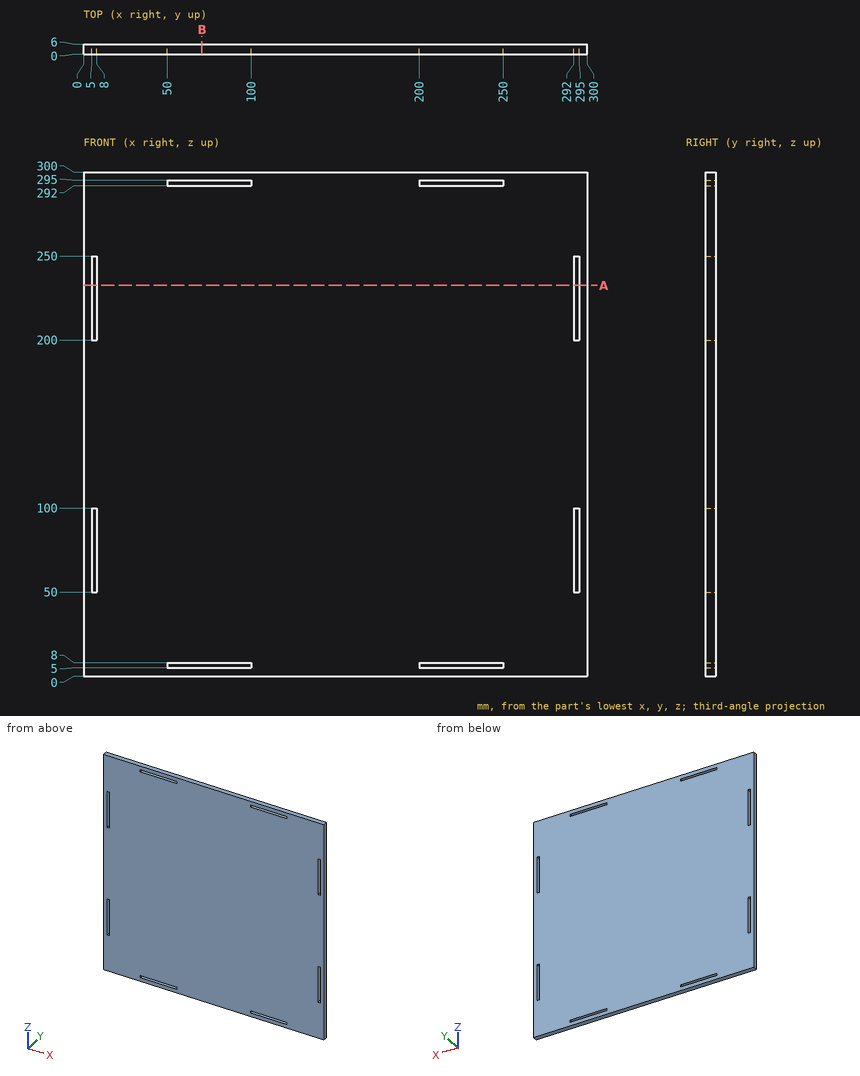
Study the drawing (mm; zero at the part's minimum x, y, z) and answer. Coordinates: 2 decimals unless noted, no trailing zeros. Loops run counter-clockwise (first coordinate to the right, second up) from the corner with the lowest first, then second, coordinate; pieces in that order, holes last. Notation, with made-up numbers: M -28,78 L -14,78 A21 cw -14,116 Z; hole C 17.5,-17.75 d6. An arc over 180 degrees is marked long. Answer as a JSON object with one key per item and string values. Group by question number.
Item 1: Section B-B (x = 70.5) is taken. Write down the section's boundary in (y, z), and give its area (3 significant figures).
Item 2: Section A-A (z = 232.5) is taken. Write down the section's boundary in (x, y).
Item 3: Consider L1, parallel to Z at x = 87.5, y = 1.4. Determine where the line is inside the solid, lowest interval first.
Solved:
{
 "1": {"outline": "M 0,0 L 6,0 L 6,5 L 0,5 Z; M 0,8 L 6,8 L 6,292 L 0,292 Z; M 0,295 L 6,295 L 6,300 L 0,300 Z", "area": "1,760 mm2"},
 "2": {"outline": "M 0,0 L 5,0 L 5,6 L 0,6 Z; M 8,0 L 292,0 L 292,6 L 8,6 Z; M 295,0 L 300,0 L 300,6 L 295,6 Z"},
 "3": {"L1": "z = 0 to 5, 8 to 292, 295 to 300"}
}
